Read the model definition and answer for the solid it produces. Units are mm, in the model's axes. Face numbers are marked on the shaded views. Give positions to 0.01 mm unless a question says otherwise; leave off trailing zeros. Loops run counter-clockwise (first coordinate to the right, second up) from the corner with the lowest first, then second, coordinate; pieces in that order, holes last. Notation, with made-up numbers: (-20, 86.25) -> (10, 86.25) arc R30 ccw to (10, 108.25) -> close; hole circle Ø5 at (36.25, -10.75). An arc over 180 degrees is marked (long way). Return JSON: item names as keys, results as strings. Group by question number.
Autodesk Inventor part; units mm, degrees
ref_plane "Mittelebene - PCB-Dicke" through (-1, 0, 0) normal (1, 0, 0) x (0, 1, 0)
ref_plane "XZ Plane" through (0, 0, 0) normal (0, 1, 0) x (-1, 0, 0)
ref_plane "XY Plane" through (0, 0, 0) normal (0, 0, 1) x (1, 0, 0)
sketch "Skizze1" plane through (0, 0, 0) normal (0, 0, 1) x (1, 0, 0)
  circle A0 centre (0, 0) radius 4
  dimension "d0" = 8
extrude "Extrusion1" add sketch "Skizze1" along normal blind 45
ref_plane "Mittelebene" through (0, 0, 0) normal (1, 0, 0) x (0, 1, 0)
ref_plane "Mittelebene - PCB-Dicke" through (-1, 0, 0) normal (1, 0, 0) x (0, 1, 0)
sketch "Skizze8" plane through (0, 0, 0) normal (1, 0, 0) x (0, 1, 0)
  line L0 (-4, 45) -> (4, 45)
  line L1 (4, 45) -> (4, 6)
  line L2 (4, 6) -> (-4, 6)
  line L3 (-4, 6) -> (-4, 45)
  point P0 (0, 0)
  dimension "d100" = 8
  dimension "d101" = 39
extrude "Extrusion6" cut sketch "Skizze8" along normal blind 14.5
sketch "Skizze12" plane through (-1, 0, 0) normal (1, 0, 0) x (0, 1, 0)
  line L0 (2.1, 10) -> (-2.1, 10)
  line L1 (-2.1, 10) -> (-2.1, 45)
  line L2 (-2.1, 45) -> (2.1, 45)
  line L3 (2.1, 45) -> (2.1, 10)
  point P0 (0, 0)
  dimension "d103" = 4.2
  dimension "d104" = 35
extrude "Extrusion8" cut sketch "Skizze12" along normal blind 6.75
sketch "Skizze13" plane through (-1, 0, 0) normal (1, 0, 0) x (0, 1, 0)
  line L0 (3.1, 10) -> (-3.1, 10)
  line L1 (-3.1, 10) -> (-3.1, 41.2)
  line L2 (-3.1, 41.2) -> (3.1, 41.2)
  line L3 (3.1, 41.2) -> (3.1, 10)
  point P0 (0, 0)
  dimension "d105" = 6.2
  dimension "d106" = 31.2
extrude "Extrusion9" cut sketch "Skizze13" along normal blind 6.25
sketch "Skizze14" plane through (-1, 0, 0) normal (1, 0, 0) x (0, 1, 0)
  point P0 (0, 0)
  point P1 (-2, 35)
  point P2 (2, 35)
hole "Bohrung3" at (-1, -2, 35) at (-1, 2, 35) direction (-1, 0, 0) diameter 1 end through all
thread "Gewinde5"
thread "Gewinde6"
sketch "Skizze15" plane through (0, 0, 0) normal (0, 0, -1) x (-1, 0, 0)
  circle A0 centre (0, 0) radius 4
  dimension "d78" = 8
extrude "Extrusion12" add sketch "Skizze15" along normal blind 5
hole "Bohrung5" at (0, 0, 0) direction (0, 0, -1) diameter 6 end through all
hole "Bohrung6" at (0, 0, 0) direction (0, 0, 1) diameter 6 depth 15 tip angle 118
sketch "Skizze16" plane through (0, 0, -5) normal (0, 0, -1) x (-1, 0, 0)
  circle A0 centre (0, 0) radius 4
  circle A1 centre (0, 0) radius 3.5
  dimension "d95" = 7
extrude "Extrusion13" cut sketch "Skizze16" against normal blind 10
thread "Gewinde7"
fillet "Rundung1" radius 1 1 edges at (-0.5, -3.1, 41.2)
fillet "Rundung2" radius 1 1 edges at (-0.5, 3.1, 41.2)
sketch "Skizze17" plane through (-1, 0, 0) normal (1, 0, 0) x (0, 0, -1)
  line L0 (-19, -3) -> (-28, -3)
  line L1 (-28, -3) -> (-28, 3)
  line L2 (-28, 3) -> (-19, 3)
  line L3 (-19, 3) -> (-19, -3)
  point P0 (0, 0)
  dimension "d114" = 9
  dimension "d115" = 6
extrude "Extrusion14" cut sketch "Skizze17" against normal blind 1
fillet "Rundung6" radius 1 4 edges at (-1.5, -3, 19) (-1.5, 3, 19) (-1.5, 3, 28) (-1.5, -3, 28)
properties part number "PEEK-PCB-holder" material "Polyaryletherketon-Kunststoff"
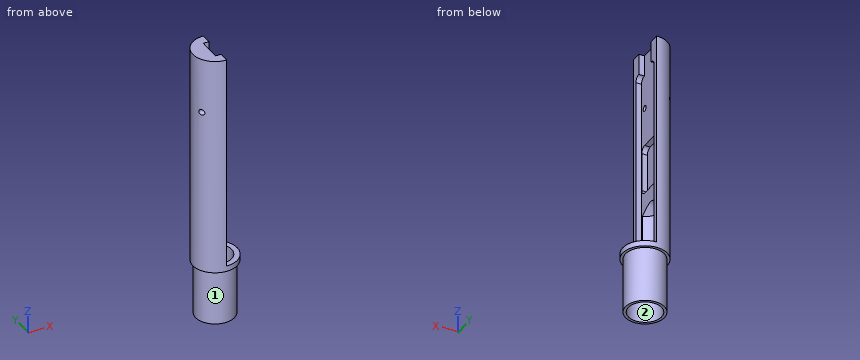
1. Determine the mould class of the marked faces 1 and 2 for opening direction Y: pulls with the +Y half, pulls with the -Y half, needs draft (parallel to the pull), parting line crosses it, or undercut.
2. Section B-B on z = 12 is taken. Determine the outline of the cut face in (x, y).
3. Section C-C on z = 35 is taken. Determine the outline of the cut face in (x, y), then the cut area to 3 significant figures.
4. Flat-ended cylindrical pins translate along their axes: pin 1 Ø0.5 at (x, z) = (-1.5, 24.5) entering from +Y; pin 2 Ø4.5 at (x, y) = (3, -1.5) entering from +Z; pin 3 Ø2 at (y, z) = (2.5, 14.5) entering from -X. Find the tip coordinate at first contact, or state that the pin passes through.
5. Straight lines are drawn through the part: line 1 (Z direction, x = -3.05, y = 2); line 2 (Z direction, x = -2.4, y = 2); line 3 (Y direction, x = -2.8, z = 35). For each, find the intervals that lie inside material, in ascending order. Write a range as from..to.
6. Section D-D on z = 1 is taken. Determine the outline of the cut face in (x, y).
7. Section A-A on x = 1.75 is taken. Determine the outline of the cut face in (y, z).
Completed:
{
 "1": {"face 1": "parting line crosses it", "face 2": "undercut"},
 "2": {"outline": "(-1, -3.1) -> (-1, -2.83) arc R3 cw to (-1, 2.83) -> (-1, 3.1) -> (0, 3.1) -> (0, 4) arc R4 ccw to (0, -4) -> (0, -3.1) -> close"},
 "3": {"outline": "(-3.71, -1.5) -> (-1, -1.5) -> (-1, 1.5) -> (-3.71, 1.5) arc R4 ccw to start; (-3.12, -2.5) arc R4 ccw to (0, -4) -> (0, -3.1) -> (-1, -3.1) -> (-1, -2.5) -> close; (-3.12, 2.5) -> (-1, 2.5) -> (-1, 3.1) -> (0, 3.1) -> (0, 4) arc R4 ccw to start", "area": "14.0 mm²"},
 "4": {"pin 1": "stops at y = 3.8", "pin 2": "stops at z = 6", "pin 3": "stops at x = -3.71"},
 "5": {"line 1": "z = 5..34.5, 35.5..45", "line 2": "z = -5..34.5, 35.5..45", "line 3": "y = -2.86..-2.5, -1.5..1.5, 2.5..2.86"},
 "6": {"outline": "circle Ø7 at (0, 0); hole circle Ø6 at (0, 0)"},
 "7": {"outline": "(-3.6, 5) -> (-3.03, 5) -> (-3.03, -5) -> (-2.44, -5) -> (-2.44, 6) -> (-3.6, 6) -> close; (2.44, -5) -> (3.03, -5) -> (3.03, 5) -> (3.6, 5) -> (3.6, 6) -> (2.44, 6) -> close"}
}
